Work out the finished part from the listing and answer in its coordinate system (mm). A direction names the side the tool comes from. Coordinates: 2 decimals unless noted, no trailing zeros. Order: outer loops, then holes, each group sorted by start corner. A loop starts at its lowest first (then second) coordinate and runs counter-clockwise, first axis right, second up. Notation, with made-up numbers: (43, 79.5) - (73, 79.5) arc R12 ccw to (73, 87.5) - close; hole circle Ø9 at (72.5, -16.75). An arc over 180 degrees is marked (long way). Answer as a JSON object with one key per item and string values. Group by question number.
1) The mould has two halves that part along Y. Classify faces 1 (the face through (0.1, 3, 13.7)), 2 (the face through (-20, 0, 7)), 3 (the face through (-19, 19, -16)): released by +Y, released by -Y, zero draft, split by the parting line, or undercut.
2) Each of these flat-tipped pins is pushed along its axis until it touches: P1, Ø0.9, axis at y = 16, z = -17, coming from the +X side; P2, Ø4, axis at x = 10, y = 10, coming from the +Z side; P3, Ø5, axis at x = -13, z = 11.5, coming from the -Y side; P4, Ø2, axis at y = 8, z = -2, coming from the -X side. Where does it stop, or does it pass through?
3) Find the intervals of material crossed by line 1 along Y through (x, z) = (10, 2); line 2 along X through (y, z) = (13, -25.25); line 3 along Y through (x, z) = (18, 12.5), in increasing order.
4) Section C-C (y = 4) is taken. Give the vertices of the cut face in (x, z).
5) Section B-B (x = -18) is taken. Give the vertices of the cut face in (y, z).
6) Section D-D (z = -5) is taken. Give the vertices of the cut face in (x, y).
7) A tool of negligible diameter and unlimited length cuts with its end or side. For faces 4 (the face through (0, -10, 8)), 5 (the face through (-6, 25, -10.5)), 6 (the face through (-19, -3, 9)), 7 (the face through (-19.75, 0.08, 4.54)), from which of +Z, -Z, +X, -X, +Y, -Y can it reach the whole face along a straight path? Write none if from no direction.
8) Section A-A (y = 17) is taken. Give the vertices of the cut face in (x, z), plus the area to 3 significant figures.
from build123d import *

# Parameters (mm, degrees)
F0_W      = 45
F0_H      = 27
F0_R      = 1.75
F0_H_2    = 14.5
F1_DEPTH  = 8
F2_DEPTH  = 28
F3_W      = 31
F3_H      = 12
F4_DEPTH  = 10
F6_DEPTH  = 19.501
F7_DEPTH  = 3
F8_R      = 8
F9_DEPTH  = 3
F11_DEPTH = 11
F12_DEPTH = 8
F13_R     = 1.75
F14_DEPTH = 16
F15_W     = 12
F15_H     = 12
F16_DEPTH = 41.501
F17_DEPTH = 17.5
F18_R     = 1.75
F19_DEPTH = 17.5
F20_W     = 6
F20_H     = 3
F21_DEPTH = 41.501
F22_R     = 5


with BuildPart() as f1:
    # F0 (on Top) → F1 (new body)
    with BuildSketch(Plane.XY):
        Rectangle(F0_W, F0_H)
        with Locations((-10, -10)):
            Circle(F0_R, mode=Mode.SUBTRACT)
        with Locations((10, -10)):
            Circle(F0_R, mode=Mode.SUBTRACT)
        with Locations((-10, 10)):
            Circle(F0_R, mode=Mode.SUBTRACT)
        with Locations((10, 10)):
            Circle(F0_R, mode=Mode.SUBTRACT)
        with Locations((0, 20.75)):
            Rectangle(F0_W, F0_H_2)
    extrude(amount=F1_DEPTH)

    # F0 (on Top) → F2 (join)
    with BuildSketch(Plane.XY):
        with Locations((0, 20.75)):
            Rectangle(F0_W, F0_H_2)
    extrude(amount=-F2_DEPTH)

    # F3 (on face) → F4 (join)
    with BuildSketch(Plane.XY.offset(8)):
        Polygon((-22.5, 28), (-22.5, -6), (-15.5, -6), (-15.5, 6), (-15.5, 28), align=None)
        Rectangle(F3_W, F3_H)
        Polygon((15.5, 6), (15.5, -6), (22.5, -6), (22.5, 28), (15.5, 28), align=None)
    extrude(amount=F4_DEPTH)

    # F5 (on face) → F6 (cut, through all)
    with BuildSketch(Plane(origin=(0, 6, 0), x_dir=(-1, 0, 0), z_dir=(0, 1, 0))):
        with BuildLine():
            Line((5.6568542495, 18), (-5.6568542495, 18))
            ThreePointArc((-5.6568542495, 18), (0, 14), (5.6568542495, 18))
        make_face()
    extrude(amount=-F6_DEPTH, mode=Mode.SUBTRACT)

    # F5 (on face) → F7 (cut)
    with BuildSketch(Plane(origin=(0, 6, 0), x_dir=(-1, 0, 0), z_dir=(0, 1, 0))):
        with BuildLine():
            Line((-5.6568542495, 18), (-7.7459666924, 18))
            ThreePointArc((-7.7459666924, 18), (0, 12), (7.7459666924, 18))
            Line((7.7459666924, 18), (5.6568542495, 18))
            ThreePointArc((5.6568542495, 18), (0, 14), (-5.6568542495, 18))
        make_face()
    extrude(amount=-F7_DEPTH, mode=Mode.SUBTRACT)

    # F8 (on face) → F9 (cut)
    with BuildSketch(Plane.XZ.offset(6)):
        with Locations((0, 20)):
            Circle(F8_R)
    extrude(amount=-F9_DEPTH, mode=Mode.SUBTRACT)

    # F10 (on face) → F11 (cut)
    with BuildSketch(Plane.XY.offset(18)):
        Polygon((-19.7320508076, -3), (-16.2679491924, -3), (-14.5358983849, 0), (-16.2679491924, 3), (-19.7320508076, 3), (-22.5, 3), (-22.5, -3), align=None)
        Polygon((14.5358983849, 0), (16.2679491924, -3), (19.7320508076, -3), (22.5, -3), (22.5, 3), (19.3412657973, 3), (16.2679491924, 3), align=None)
    extrude(amount=-F11_DEPTH, mode=Mode.SUBTRACT)

    # F10 (on face) → F12 (join)
    with BuildSketch(Plane.XY.offset(18)):
        Polygon((-19.7320508076, -3), (-16.2679491924, -3), (-14.5358983849, 0), (-16.2679491924, 3), (-19.7320508076, 3), (-22.5, 3), (-22.5, -3), align=None)
        Polygon((14.5358983849, 0), (16.2679491924, -3), (19.7320508076, -3), (22.5, -3), (22.5, 3), (19.3412657973, 3), (16.2679491924, 3), align=None)
    extrude(amount=-F12_DEPTH)

    # F13 (on face) → F14 (cut)
    with BuildSketch(Plane.XY.offset(18)):
        with Locations((-18, 0)):
            Circle(F13_R)
        with Locations((18, 0)):
            Circle(F13_R)
    extrude(amount=-F14_DEPTH, mode=Mode.SUBTRACT)

    # F15 (on face) → F16 (cut, through all)
    with BuildSketch(Plane(origin=(0, 28, 0), x_dir=(-1, 0, 0), z_dir=(0, 1, 0))):
        with Locations((16.5, -22)):
            Rectangle(F15_W, F15_H)
        with Locations((-16.5, -22)):
            Rectangle(F15_W, F15_H)
    extrude(amount=-F16_DEPTH, mode=Mode.SUBTRACT)

    # F15 (on face) → F17 (join)
    with BuildSketch(Plane(origin=(0, 28, 0), x_dir=(-1, 0, 0), z_dir=(0, 1, 0))):
        Polygon((-10.5, -16), (-10.5, -28), (10.5, -28), (10.5, -16), (22.5, -16), (22.5, -10.5), (-22.5, -10.5), (-22.5, -16), align=None)
    extrude(amount=-F17_DEPTH)

    # F18 (on face) → F19 (cut)
    with BuildSketch(Plane(origin=(0, 0, -28), x_dir=(1, 0, 0), z_dir=(0, 0, -1))):
        with Locations((-6, -13)):
            Circle(F18_R)
        with Locations((6, -13)):
            Circle(F18_R)
        with Locations((6, -25)):
            Circle(F18_R)
        with Locations((-6, -25)):
            Circle(F18_R)
    extrude(amount=-F19_DEPTH, mode=Mode.SUBTRACT)

    # F20 (on face) → F21 (cut, through all)
    with BuildSketch(Plane(origin=(0, 28, 0), x_dir=(-1, 0, 0), z_dir=(0, 1, 0))):
        with Locations((-6, -17.5)):
            Rectangle(F20_W, F20_H)
        with Locations((6, -17.5)):
            Rectangle(F20_W, F20_H)
    extrude(amount=-F21_DEPTH, mode=Mode.SUBTRACT)

    # F22
    f22_edges = [f1.edges().sort_by_distance(p)[0] for p in [
        (-10.5, 19.25, -16),
        (10.5, 19.25, -16),
    ]]
    fillet(f22_edges, radius=F22_R)


solid = f1.part
Report:
{
 "1": {"face 1": "released by +Y", "face 2": "undercut", "face 3": "zero draft"},
 "2": {"P1": "stops at x = 13.22", "P2": "stops at z = 8", "P3": "stops at y = -6", "P4": "passes through"},
 "3": {"line 1": "y = -13.5 to -11.75, -8.25 to 8.25, 11.75 to 28", "line 2": "x = -10.5 to -7.75, -4.25 to 4.25, 7.75 to 10.5", "line 3": "y = -6 to -1.75, 1.75 to 28"},
 "4": {"outline": "(-22.5, 0) - (22.5, 0) - (22.5, 18) - (7.75, 18) arc R8 cw to (-7.75, 18) - (-22.5, 18) - close"},
 "5": {"outline": "(-13.5, 0) - (13.5, 0) - (13.5, -10.5) - (10.5, -10.5) - (10.5, -16) - (28, -16) - (28, 18) - (1.75, 18) - (1.75, 10) - (3, 10) - (3, 7) - (1.75, 7) - (1.75, 2) - (-1.75, 2) - (-1.75, 7) - (-3, 7) - (-3, 10) - (-1.75, 10) - (-1.75, 18) - (-6, 18) - (-6, 8) - (-13.5, 8) - close"},
 "6": {"outline": "(-22.5, 13.5) - (22.5, 13.5) - (22.5, 28) - (-22.5, 28) - close"},
 "7": {"face 4": "+Z, +X, -X, -Y", "face 5": "-Z", "face 6": "-X", "face 7": "+Z"},
 "8": {"outline": "(-22.5, -16) - (-15.5, -16) arc R5 cw to (-10.5, -21) - (-10.5, -28) - (10.5, -28) - (10.5, -21) arc R5 cw to (15.5, -16) - (22.5, -16) - (22.5, 18) - (15.5, 18) - (15.5, 8) - (-15.5, 8) - (-15.5, 18) - (-22.5, 18) - close; hole (-9, -19) - (-3, -19) - (-3, -16) - (-9, -16) - close; hole (3, -19) - (9, -19) - (9, -16) - (3, -16) - close", "area": "1,450 mm²"}
}
